```python
from build123d import *

# Parameters (mm, degrees)
F0_R     = 11.08
F1_DEPTH = 7
F2_R     = 25


with BuildPart() as f1:
    # F0 (on Top) → F1 (new body)
    with BuildSketch(Plane.XY):
        with BuildLine():
            ThreePointArc((2.6624965293, 34.2446519242), (3.3990862891, 31.8515325068), (4.1848381854, 29.4741013348))
            ThreePointArc((4.1848381854, 29.4741013348), (8.2251664175, 31.1828715934), (11.6533257056, 33.92))
            ThreePointArc((11.6533257056, 33.92), (14.9323788685, 39.0342258401), (16.08, 45))
            ThreePointArc((16.08, 45), (-5.9657741599, 59.9323788685), (-11.6533257056, 33.92))
            ThreePointArc((-11.6533257056, 33.92), (-8.2251664175, 31.1828715934), (-4.1848381854, 29.4741013348))
            ThreePointArc((-4.1848381854, 29.4741013348), (-3.3990862891, 31.8515325068), (-2.6624965293, 34.2446519242))
            ThreePointArc((-2.6624965293, 34.2446519242), (-6.8288336653, 53.7254473107), (11.08, 45))
            ThreePointArc((11.08, 45), (8.7254473107, 38.1711663347), (2.6624965293, 34.2446519242))
        make_face()
        with BuildLine():
            ThreePointArc((-11.6533257056, 33.92), (-9.9229010426, 20.728301046), (-13.9256884929, 8.04))
            ThreePointArc((-13.9256884929, 8.04), (-8.5348333079, 18.5205382543), (-4.1848381854, 29.4741013348))
            ThreePointArc((-4.1848381854, 29.4741013348), (-8.2251664175, 31.1828715934), (-11.6533257056, 33.92))
        make_face()
        with BuildLine():
            ThreePointArc((-4.1848381854, 29.4741013348), (0, 28.92), (4.1848381854, 29.4741013348))
            ThreePointArc((4.1848381854, 29.4741013348), (3.3990862891, 31.8515325068), (2.6624965293, 34.2446519242))
            ThreePointArc((2.6624965293, 34.2446519242), (0, 33.92), (-2.6624965293, 34.2446519242))
            ThreePointArc((-2.6624965293, 34.2446519242), (-3.3990862891, 31.8515325068), (-4.1848381854, 29.4741013348))
        make_face()
        with BuildLine():
            ThreePointArc((-13.9256884929, 8.04), (0, 16.08), (13.9256884929, 8.04))
            ThreePointArc((13.9256884929, 8.04), (8.5348333079, 18.5205382543), (4.1848381854, 29.4741013348))
            ThreePointArc((4.1848381854, 29.4741013348), (0, 28.92), (-4.1848381854, 29.4741013348))
            ThreePointArc((-4.1848381854, 29.4741013348), (-8.5348333079, 18.5205382543), (-13.9256884929, 8.04))
        make_face()
        with BuildLine():
            ThreePointArc((4.1848381854, 29.4741013348), (8.5348333079, 18.5205382543), (13.9256884929, 8.04))
            ThreePointArc((13.9256884929, 8.04), (9.9229010426, 20.728301046), (11.6533257056, 33.92))
            ThreePointArc((11.6533257056, 33.92), (8.2251664175, 31.1828715934), (4.1848381854, 29.4741013348))
        make_face()
        with BuildLine():
            ThreePointArc((-22.8911431703, -22.5), (-23.0271579816, -20.4129599182), (-23.4329014169, -18.3612268467))
            ThreePointArc((-23.4329014169, -18.3612268467), (-25.8846931558, -18.8694613295), (-28.3254902455, -19.4281155939))
            ThreePointArc((-28.3254902455, -19.4281155939), (-28.0002673072, -20.948780223), (-27.8911431703, -22.5))
            ThreePointArc((-27.8911431703, -22.5), (-49.247810258, -26.6420421978), (-30.9879867747, -14.8165363303))
            ThreePointArc((-30.9879867747, -14.8165363303), (-29.2837794449, -12.9820711774), (-27.6177396024, -11.1128744881))
            ThreePointArc((-27.6177396024, -11.1128744881), (-31.1177421715, -8.4682327288), (-35.2022445492, -6.8679239004))
            ThreePointArc((-35.2022445492, -6.8679239004), (-52.8968316632, -30.54), (-23.5489188436, -27.0520760996))
            ThreePointArc((-23.5489188436, -27.0520760996), (-23.0564366513, -24.7996774585), (-22.8911431703, -22.5))
        make_face()
        with BuildLine():
            ThreePointArc((-28.3254902455, -19.4281155939), (-25.8846931558, -18.8694613295), (-23.4329014169, -18.3612268467))
            ThreePointArc((-23.4329014169, -18.3612268467), (-25.0454546774, -14.46), (-27.6177396024, -11.1128744881))
            ThreePointArc((-27.6177396024, -11.1128744881), (-29.2837794449, -12.9820711774), (-30.9879867747, -14.8165363303))
            ThreePointArc((-30.9879867747, -14.8165363303), (-29.3755816964, -16.96), (-28.3254902455, -19.4281155939))
        make_face()
        with BuildLine():
            ThreePointArc((-27.6177396024, -11.1128744881), (-20.3066732739, -1.8688866654), (-13.9256884929, 8.04))
            ThreePointArc((-13.9256884929, 8.04), (-22.9126858044, -1.7706661409), (-35.2022445492, -6.8679239004))
            ThreePointArc((-35.2022445492, -6.8679239004), (-31.1177421715, -8.4682327288), (-27.6177396024, -11.1128744881))
        make_face()
        with BuildLine():
            ThreePointArc((-23.4329014169, -18.3612268467), (-11.771839966, -16.6516515888), (0, -16.08))
            ThreePointArc((0, -16.08), (-13.9256884929, -8.04), (-13.9256884929, 8.04))
            ThreePointArc((-13.9256884929, 8.04), (-20.3066732739, -1.8688866654), (-27.6177396024, -11.1128744881))
            ThreePointArc((-27.6177396024, -11.1128744881), (-25.0454546774, -14.46), (-23.4329014169, -18.3612268467))
        make_face()
        with BuildLine():
            ThreePointArc((-23.5489188436, -27.0520760996), (-12.9897847619, -18.9576349051), (0, -16.08))
            ThreePointArc((0, -16.08), (-11.771839966, -16.6516515888), (-23.4329014169, -18.3612268467))
            ThreePointArc((-23.4329014169, -18.3612268467), (-23.0271579816, -20.4129599182), (-22.8911431703, -22.5))
            ThreePointArc((-22.8911431703, -22.5), (-23.0564366513, -24.7996774585), (-23.5489188436, -27.0520760996))
        make_face()
        with BuildLine():
            ThreePointArc((13.9256884929, 8.04), (15.5320872867, 4.1618102452), (16.08, 0))
            ThreePointArc((16.08, 0), (11.3702770415, -11.3702770415), (0, -16.08))
            ThreePointArc((0, -16.08), (11.771839966, -16.6516515888), (23.4329014169, -18.3612268467))
            ThreePointArc((23.4329014169, -18.3612268467), (25.0454546774, -14.46), (27.6177396024, -11.1128744881))
            ThreePointArc((27.6177396024, -11.1128744881), (20.3066732739, -1.8688866654), (13.9256884929, 8.04))
        make_face()
        with BuildLine():
            ThreePointArc((23.4329014169, -18.3612268467), (11.771839966, -16.6516515888), (0, -16.08))
            ThreePointArc((0, -16.08), (12.9897847619, -18.9576349051), (23.5489188436, -27.0520760996))
            ThreePointArc((23.5489188436, -27.0520760996), (22.8925757541, -22.7146388646), (23.4329014169, -18.3612268467))
        make_face()
        with BuildLine():
            ThreePointArc((35.2022445492, -6.8679239004), (22.9126858044, -1.7706661409), (13.9256884929, 8.04))
            ThreePointArc((13.9256884929, 8.04), (20.3066732739, -1.8688866654), (27.6177396024, -11.1128744881))
            ThreePointArc((27.6177396024, -11.1128744881), (31.1177421715, -8.4682327288), (35.2022445492, -6.8679239004))
        make_face()
        with BuildLine():
            ThreePointArc((35.2022445492, -6.8679239004), (31.1177421715, -8.4682327288), (27.6177396024, -11.1128744881))
            ThreePointArc((27.6177396024, -11.1128744881), (29.2837794449, -12.9820711774), (30.9879867747, -14.8165363303))
            ThreePointArc((30.9879867747, -14.8165363303), (43.1131853681, -12.2233329123), (50.0511431703, -22.5))
            ThreePointArc((50.0511431703, -22.5), (37.4199233933, -33.4708758631), (28.3254902455, -19.4281155939))
            ThreePointArc((28.3254902455, -19.4281155939), (25.8846931558, -18.8694613295), (23.4329014169, -18.3612268467))
            ThreePointArc((23.4329014169, -18.3612268467), (22.8925757541, -22.7146388646), (23.5489188436, -27.0520760996))
            ThreePointArc((23.5489188436, -27.0520760996), (41.2708206288, -38.414706519), (55.0511431703, -22.5))
            ThreePointArc((55.0511431703, -22.5), (48.9200755294, -9.86729859), (35.2022445492, -6.8679239004))
        make_face()
        with BuildLine():
            ThreePointArc((30.9879867747, -14.8165363303), (29.2837794449, -12.9820711774), (27.6177396024, -11.1128744881))
            ThreePointArc((27.6177396024, -11.1128744881), (25.0454546774, -14.46), (23.4329014169, -18.3612268467))
            ThreePointArc((23.4329014169, -18.3612268467), (25.8846931558, -18.8694613295), (28.3254902455, -19.4281155939))
            ThreePointArc((28.3254902455, -19.4281155939), (29.3755816964, -16.96), (30.9879867747, -14.8165363303))
        make_face()
        with BuildLine():
            ThreePointArc((0, -16.08), (11.3702770415, -11.3702770415), (16.08, 0))
            ThreePointArc((16.08, 0), (15.5320872867, 4.1618102452), (13.9256884929, 8.04))
            ThreePointArc((13.9256884929, 8.04), (0, 16.08), (-13.9256884929, 8.04))
            ThreePointArc((-13.9256884929, 8.04), (-13.9256884929, -8.04), (0, -16.08))
        make_face()
        Circle(F0_R, mode=Mode.SUBTRACT)
    extrude(amount=F1_DEPTH)

    # F2
    f2_edges = [f1.edges().sort_by_distance(p)[0] for p in [
        (11.653326, 33.92, 3.5),
        (-11.653326, 33.92, 3.5),
        (35.202245, -6.867924, 3.5),
        (23.548919, -27.052076, 3.5),
        (-23.548919, -27.052076, 3.5),
        (-35.202245, -6.867924, 3.5),
    ]]
    fillet(f2_edges, radius=F2_R)


solid = f1.part
```
Geometry: final body of the model. Coordinates: model frame, mm. Coordinates: 2 decimals unless noted, no trailing zeros. Order: outer loops, then holes, each group sorted by start corner. A loop starts at its lowest first (then second) coordinate and runs counter-clockwise, first axis right, second up.
Item 1: Section query A-A (y = 0). Output: boundary loops of the cut face in (x, z), then the cut area to 3 significant figures.
Answer:
outline: (-20.62, 0) - (-11.08, 0) - (-11.08, 7) - (-20.62, 7) - close; (11.08, 0) - (20.62, 0) - (20.62, 7) - (11.08, 7) - close
area: 134 mm2
Item 2: Draft query along X for faces 1 (the face through (-53.13, -30.12, 3.45)), 2 (the face through (52.65, -30.95, 3.45)), 3 (the face through (4, -11, 7)). Return one class per face: released by +X, released by -X, zero draft, split by the parting line, or undercut.
Answer:
face 1: undercut
face 2: undercut
face 3: zero draft
Item 3: Contact query for flat-ended pins moving along their axis: P1, Ø20, axis at x = 38.97, y = -22.5, coming from the -Z side; P2, Ø1, axis at x = -14, z = 5.5, coming from the +Y side; P3, Ø3, axis at y = -1, z = 2, coming from the -X side; P4, Ø1.5, axis at y = 1, z = 3.5, coming from the +X side. Output: stop coordinate, or through.
Answer:
P1: passes through
P2: stops at y = 53.74
P3: stops at x = -24
P4: stops at x = 20.33
Item 4: Material intervals for line 1 along Y through (x, z) = (0, 3.75); line 2 along X through (y, z) = (45.5, 1); line 3 along X through (y, z) = (-22.5, 6.5), sorted ascending.
Answer:
line 1: y = -16.08 to -11.08, 11.08 to 33.92, 56.08 to 61.08
line 2: x = -16.07 to -11.07, 11.07 to 16.07
line 3: x = -55.05 to -50.05, -27.89 to -18.64, 18.64 to 27.89, 50.05 to 55.05
Item 5: Section query D-D (z = 2.25). State how many separate pieces and enclosed holes the cut face has, then the cut area to 3 significant figures.
Answer:
separate pieces: 1
enclosed holes: 4
area: 2,690 mm2
Item 6: Section query B-B (x = 44). Output: boundary loops of the cut face in (y, z), then the cut area to 3 significant figures.
Answer:
outline: (-37.77, 0) - (-32.37, 0) - (-32.37, 7) - (-37.77, 7) - close; (-12.63, 0) - (-7.23, 0) - (-7.23, 7) - (-12.63, 7) - close
area: 75.6 mm2
Item 7: Section query C-C (y = 14). Output: boundary loops of the cut face in (x, z), then the cut area to 3 significant figures.
Answer:
outline: (-11.28, 0) - (11.28, 0) - (11.28, 7) - (-11.28, 7) - close
area: 158 mm2
